Autodesk Inventor part; units mm, degrees
ref_plane "YZ Plane" through (0, 0, 0) normal (1, 0, 0) x (0, 1, 0)
ref_plane "XZ Plane" through (0, 0, 0) normal (0, 1, 0) x (-1, 0, 0)
ref_plane "XY Plane" through (0, 0, 0) normal (0, 0, 1) x (1, 0, 0)
sketch "Sketch1" plane through (0, 0, 0) normal (0, 1, 0) x (-1, 0, 0)
  line L0 (0, 62) -> (0, 57.25) construction
  line L1 (0, 62) -> (-4.75, 62) construction
  line L2 (0, -62) -> (-4.75, -62) construction
  line L3 (-117.25, -57) -> (-9.75, -57)
  line L4 (-5, -57) -> (-5, -52.25) construction
  line L5 (-5, 57) -> (-9.75, 57) construction
  line L6 (-117.25, 57) -> (-117.25, 62)
  line L7 (-117.25, -62) -> (-117.25, -57)
  arc A0 (-5, 52.25) -> (-9.75, 57) centre (-9.75, 52.25) ccw
  arc A1 (-9.75, -57) -> (-5, -52.25) centre (-9.75, -52.25) ccw
  arc A2 (0, 57.25) -> (-4.75, 62) centre (-4.75, 57.25) ccw
  arc A3 (-4.75, -62) -> (0, -57.25) centre (-4.75, -57.25) ccw
  line L8 (0, 57.25) -> (0, -57.25)
  line L9 (-4.75, 62) -> (-117.25, 62)
  line L10 (0, -57.25) -> (0, -62) construction
  line L11 (-4.75, -62) -> (-117.25, -62)
  line L12 (-5, -52.25) -> (-5, 52.25)
  line L13 (-9.75, -57) -> (-5, -57) construction
  line L14 (-5, 52.25) -> (-5, 57) construction
  line L15 (-9.75, 57) -> (-117.25, 57)
  arc A4 (-4.75, 62) -> (0, 57.25) centre (-4.75, 57.25) ccw construction
  arc A5 (-9.75, 57) -> (-5, 52.25) centre (-9.75, 52.25) ccw construction
  arc A6 (0, -57.25) -> (-4.75, -62) centre (-4.75, -57.25) ccw construction
  arc A7 (-5, -52.25) -> (-9.75, -57) centre (-9.75, -52.25) ccw construction
  point P0 (0, 0)
  point P1 (0, 0)
  dimension "d4" = 5
  dimension "d6" = 117.25
  dimension "d8" = 117.25
  dimension "d9" = 5
  dimension "d10" = 5
  dimension "d11" = 124
  dimension "d12" = 57
  dimension "d14" = 9.5
extrude "Plate1" add sketch "Sketch1" against normal blind 2
equation "\"d9\" = d4"
equation "\"d10\" = d4"
equation "\"d11\" = Ширина_крепления_корпуса + 2 * Thickness"
equation "\"d5\" = Thickness"
equation "\"BendReliefWidth\" = Thickness"
equation "\"BendReliefDepth\" = 0.5 * Thickness"
equation "\"CornerReliefSize\" = 4 * Thickness"
equation "\"MinimumRemnant\" = 2 * Thickness"
equation "\"TransitionRadius\" = BendRadius"
equation "\"JacobiRadiusSize\" = BendRadius"
equation "\"GapSize\" = Thickness"
properties part number "Опоры на кожухе" material "Stainless Steel"
Model file for the job. Use its own axes, mm. A direction names the side the tool comes from. Give positions to 0.01 mm unless a question says otherwise; leave off trailing zeros. Order: outer loops, then holes, each group sorted by start corner. A loop starts at its lowest first (then second) coordinate and runs counter-clockwise, first axis right, second up. Notation, with made-up numbers: M 30.5,-15.75 L 68.5,-15.75 A18 cw 68.5,18.25 Z; hole C 0,41 d5. An arc over 180 degrees is marked long. Put each result on its own line as item: value. Start each with the question number.
(1) Drill centre lines: L1, parallel to Z at x = 45.5, y = -0.9; L2, parallel to X at y = -1.1, z = 40.5. Where is each one in solid material? Low to high. Write a range as [from, to].
(2) Band-saw the part on A-A on x = 70. Give the cut face in (y, z), then the cut area to 3 significant figures.
(3) Band-saw the part on B-B on y = -0.55. Give the cut face in (x, z).
(4) Band-saw the part on C-C on z = -2.5. Give the cut face in (x, y), then the cut area to 3 significant figures.
(5) Pull direction Z, two halves, no side cores. Call faces 3 (the face through (1.428, -0.986, -60.645)), 4 (the face through (1.355, -0.986, 60.572)), 5 (the face through (6.355, -0.986, 55.572)), 6 (the face through (2, -2, 0)): released by +Z, released by -Z, zero draft, split by the parting line, or undercut.
(6) Tool access for faces 1 (the face through (6.428, -0.986, -55.645)), 2 (the face through (2, 0, 0)): list every direction of +Z, -Z, +X, -X, +Y, -Y with a clear straight run to the whole face (end or side of a thin tool).
(7) Pin check, flat tip, straight feed: pin 1 Ø0.6 at (y, z) = (-1, 6) entering from +X. Stop position of the tip, or through.
Results below:
1. L1: z = [-62, -57], [57, 62]
1. L2: x = [0, 5]
2. outline: M -2,-62 L 0,-62 L 0,-57 L -2,-57 Z; M -2,57 L 0,57 L 0,62 L -2,62 Z
2. area: 20.0 mm2
3. outline: M 0,-57.25 A4.75 ccw 4.75,-62 L 117.25,-62 L 117.25,-57 L 9.75,-57 A4.75 cw 5,-52.25 L 5,52.25 A4.75 cw 9.75,57 L 117.25,57 L 117.25,62 L 4.75,62 A4.75 ccw 0,57.25 Z
4. outline: M 0,-2 L 5,-2 L 5,0 L 0,0 Z
4. area: 10.0 mm2
5. face 3: released by -Z
5. face 4: released by +Z
5. face 5: undercut
5. face 6: zero draft
6. face 1: +X, +Y, -Y
6. face 2: +Z, -Z, +X, -X, +Y
7. pin 1: stops at x = 5
